Could you check a few things on this drawing? It's one solid part, dimensions in mm from its lowest x, y, z. A direction names the side the tool comes from. Give positions to 0.01 mm unless a question says otherwise; leave off trailing zeros. Loops run counter-clockwise (first coordinate to the right, second up) from the corner with the lowest first, then second, coordinate; pieces in that order, holes last.
1. For P1, Ø1.5, axis at x = 93.5, z = 35.5, coming from the +Y side; P2, Ø3, axis at x = 68, z = 48.5, coming from the +Y side; P3, Ø1, axis at y = 11, z = 26, coming from the +X side, each with a flat end and sliding along its axis, tell me the tip position at first contact or that it passes through.
2. Imagine slicing it at D-D (x = 50). List the corners of the cut face in (y, z) for me.
3. Imagine slicing it at B-B (x = 8.6). List the corners of the cut face in (y, z) for me.
4. For the marked faces 4 and 5, which set-ups out of +Z, -Z, +X, -X, +Y, -Y let a thin tool reach every point of the face, with its end or its side?
5. Imagine slicing it at A-A (y = 16.75). List the corners of the cut face in (x, z) for me, plus the area to 3 significant figures.
6. Thinking about a two-plate mould opening in X: for the marked faces 1, 2 and 3, which applies, +X half, -X half, draft (parallel to the pull), parting line (faces both ways), or undercut?
7. Imagine slicing it at C-C (z = 38). List the corners of the cut face in (x, y) for me.
8. I need wall thicknesses on line 1 along Z through (x, y) = (33, 10.25); line 2 along Y through (x, z) = (55, 25); line 3 along Y through (x, z) = (16.5, 15). Which ranges of each line are inside material? Lowest first, please.
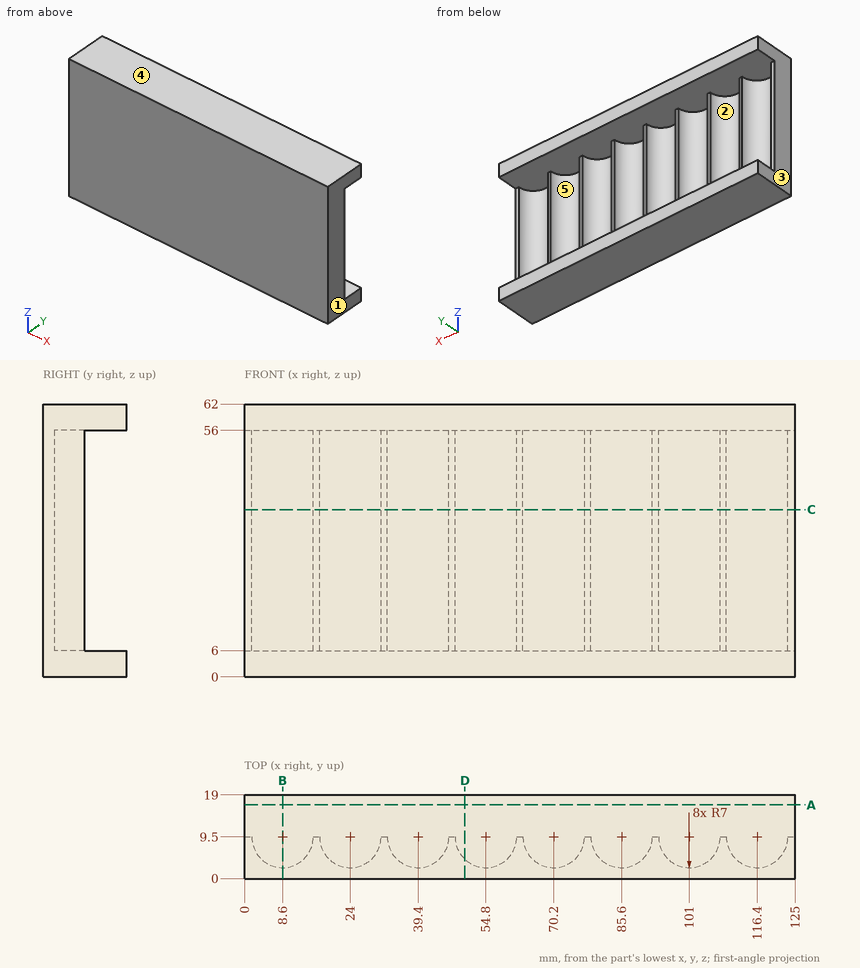
Derived:
1. P1: stops at y = 9.5
1. P2: stops at y = 3.56
1. P3: passes through
2. outline: (0, 0) - (19, 0) - (19, 6) - (4.4, 6) - (4.4, 56) - (19, 56) - (19, 62) - (0, 62) - close
3. outline: (0, 0) - (19, 0) - (19, 6) - (2.5, 6) - (2.5, 56) - (19, 56) - (19, 62) - (0, 62) - close
4. face 4: +Z, +X, -X, +Y, -Y
4. face 5: +Y
5. outline: (0, 0) - (125, 0) - (125, 6) - (0, 6) - close; (0, 56) - (125, 56) - (125, 62) - (0, 62) - close
5. area: 1,500 mm2
6. face 1: +X half
6. face 2: undercut
6. face 3: -X half
7. outline: (0, 0) - (125, 0) - (125, 9.5) - (123.4, 9.5) arc R7 cw to (109.4, 9.5) - (108, 9.5) arc R7 cw to (94, 9.5) - (92.6, 9.5) arc R7 cw to (78.6, 9.5) - (77.2, 9.5) arc R7 cw to (63.2, 9.5) - (61.8, 9.5) arc R7 cw to (47.8, 9.5) - (46.4, 9.5) arc R7 cw to (32.4, 9.5) - (31, 9.5) arc R7 cw to (17, 9.5) - (15.6, 9.5) arc R7 cw to (1.6, 9.5) - (0, 9.5) - close
8. line 1: z = 0 to 6, 56 to 62
8. line 2: y = 0 to 2.5
8. line 3: y = 0 to 9.5
